Print and shaded views of the part. All mm, measured from the part's lowest x, y and z. Give positions to 0.01 mm unless a question says otherwise; leave off trailing zeros. Loops run counter-clockwise (first coordinate to the right, second up) from the corner with the lowest first, then second, coordinate; pieces in that order, holes last.
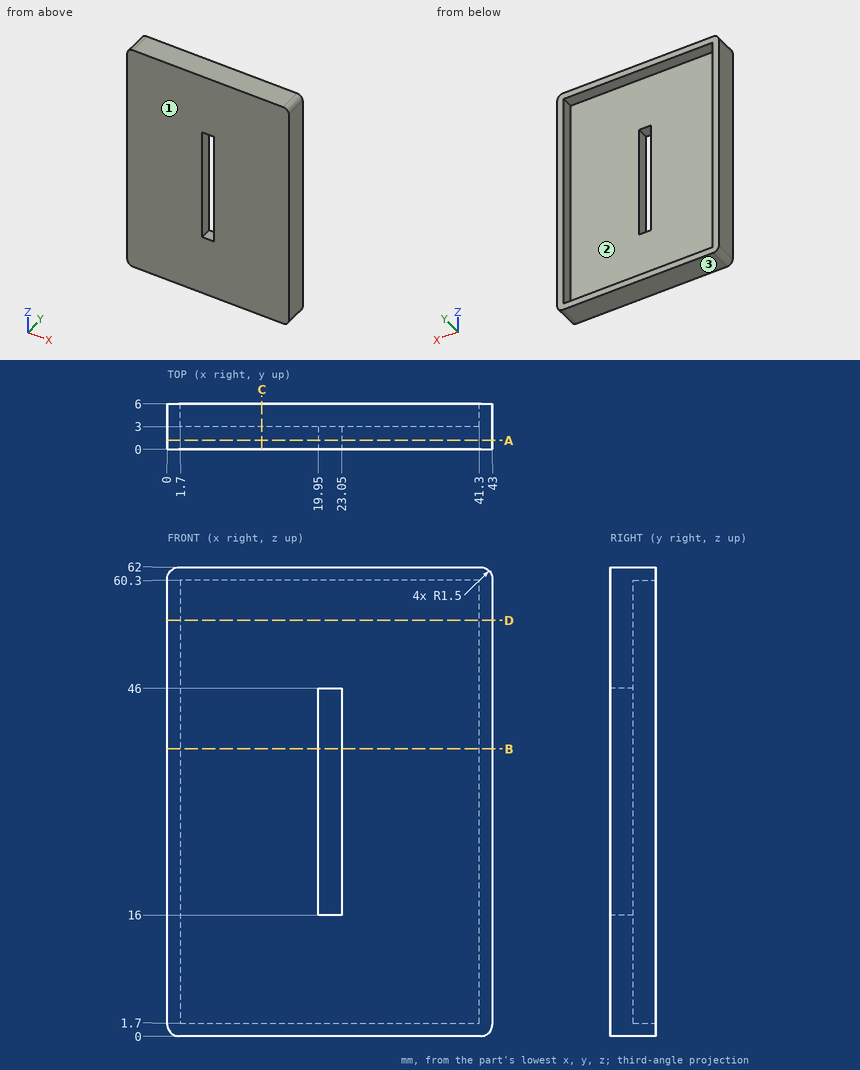
1. Saw through at D-D, the plane z = 55. List the corners of the cut face in (x, y).
Responses:
outline: (0, 0) - (43, 0) - (43, 6) - (41.3, 6) - (41.3, 3) - (1.7, 3) - (1.7, 6) - (0, 6) - close
2. Saw through at C-C, the plane x = 12.5. List the corners of the cut face in (y, z), and give its area (3 significant figures).
Responses:
outline: (0, 0) - (6, 0) - (6, 1.7) - (3, 1.7) - (3, 60.3) - (6, 60.3) - (6, 62) - (0, 62) - close
area: 196 mm2
3. Probe line 1 along Z through (x, y) = (39.5, 4.65); line 2 along X through (y, z) = (1.35, 39); line 3 along X through (y, z) = (4.45, 8). List the from-to ranges inside material, lowest first.
Responses:
line 1: z = 0 to 1.7, 60.3 to 62
line 2: x = 0 to 19.95, 23.05 to 43
line 3: x = 0 to 1.7, 41.3 to 43
4. Saw through at A-A, the plane y = 1.2. List the corners of the cut face in (x, z).
Responses:
outline: (0, 1.5) arc R1.5 ccw to (1.5, 0) - (41.5, 0) arc R1.5 ccw to (43, 1.5) - (43, 60.5) arc R1.5 ccw to (41.5, 62) - (1.5, 62) arc R1.5 ccw to (0, 60.5) - close; hole (19.95, 16) - (23.05, 16) - (23.05, 46) - (19.95, 46) - close
5. Pull direction Z, two halves, no side cores. Call the marked faces 1, 2 and 3: released by +Z, released by -Z, zero draft, split by the parting line, or undercut.
Responses:
face 1: zero draft
face 2: undercut
face 3: released by -Z
6. Saw through at B-B, the plane z = 38. List the corners of the cut face in (x, y).
Responses:
outline: (0, 0) - (19.95, 0) - (19.95, 3) - (1.7, 3) - (1.7, 6) - (0, 6) - close; (23.05, 0) - (43, 0) - (43, 6) - (41.3, 6) - (41.3, 3) - (23.05, 3) - close
7. Drop a flat-ended pin along its axis: pin 1 (12 mm diameter, centred on x = 13.5, z = 17.5, fed in from +Y). Give the stop position or say it passes through.
Responses:
pin 1: stops at y = 3
